```python
from build123d import *

# Parameters (mm, degrees)
SKETCH1_W               = 110
SKETCH1_H               = 70
BOSS_EXTRUDE1_DEPTH     = 5
FILLET2_R               = 5
FILLET3_R               = 5
SKETCH2_W               = 5
SKETCH2_H               = 10
BOSS_EXTRUDE2_DEPTH     = 10
SKETCH3_R               = 1.5
CUT_EXTRUDE1_DEPTH      = 122
SKETCH4_W               = 70
SKETCH4_H               = 10
BOSS_EXTRUDE3_DEPTH     = 10
SKETCH5_R               = 11.5
CUT_EXTRUDE2_DEPTH      = 105
SKETCH6_R               = 1.5
CUT_EXTRUDE3_DEPTH      = 105
CUT_EXTRUDE4_DEPTH      = 55
CUT_EXTRUDE4_DEPTH_BACK = 5
SKETCH9_W               = 90
SKETCH9_H               = 50
CUT_EXTRUDE5_DEPTH      = 55
SKETCH10_R              = 12
CUT_EXTRUDE6_DEPTH      = 109


with BuildPart() as part:
    # Sketch1 → Boss-Extrude1 (new body)
    with BuildSketch(Plane(origin=(0, 0, 0), x_dir=(0, 0, -1), z_dir=(1, 0, 0))):
        with Locations((55, 35)):
            Rectangle(SKETCH1_W, SKETCH1_H)
    extrude(amount=BOSS_EXTRUDE1_DEPTH)

    # Fillet2
    fillet2_edges = [part.edges().sort_by_distance(p)[0] for p in [
        (5, 35, 0),
    ]]
    fillet(fillet2_edges, radius=FILLET2_R - 0.0001)  # a hair under: the kernel refuses the full size

    # Fillet3
    fillet3_edges = [part.edges().sort_by_distance(p)[0] for p in [
        (5, 35, -110),
    ]]
    fillet(fillet3_edges, radius=FILLET3_R - 0.0001)  # a hair under: the kernel refuses the full size

    # Sketch2 → Boss-Extrude2 (add)
    with BuildSketch(Plane.ZY):
        with Locations((-102.5, 65)):
            Rectangle(SKETCH2_W, SKETCH2_H)
        with Locations((-102.5, 5)):
            Rectangle(SKETCH2_W, SKETCH2_H)
        with Locations((-7.5, 5)):
            Rectangle(SKETCH2_W, SKETCH2_H)
        with Locations((-7.5, 65)):
            Rectangle(SKETCH2_W, SKETCH2_H)
    extrude(amount=BOSS_EXTRUDE2_DEPTH)

    # Sketch3 → Cut-Extrude1 (cut)
    with BuildSketch(Plane.XY.offset(-5)):
        with Locations((-5, 65)):
            Circle(SKETCH3_R)
        with Locations((-5, 5)):
            Circle(SKETCH3_R)
    extrude(amount=-CUT_EXTRUDE1_DEPTH, mode=Mode.SUBTRACT)

    # Sketch4 → Boss-Extrude3 (add)
    with BuildSketch(Plane.ZY):
        with Locations((-55, 65)):
            Rectangle(SKETCH4_W, SKETCH4_H)
        with Locations((-55, 5)):
            Rectangle(SKETCH4_W, SKETCH4_H)
    extrude(amount=BOSS_EXTRUDE3_DEPTH)

    # Sketch5 → Cut-Extrude2 (cut)
    with BuildSketch(Plane.XY.offset(-5)):
        with Locations((-17.5, 15)):
            Circle(SKETCH5_R)
    extrude(amount=-CUT_EXTRUDE2_DEPTH, mode=Mode.SUBTRACT)

    # Sketch6 → Cut-Extrude3 (cut)
    with BuildSketch(Plane.XZ):
        with Locations(Location((-3.573842411, -25, 0), (0, 0, 270))):
            Circle(SKETCH6_R)
        with Locations(Location((-3.573842411, -85, 0), (0, 0, 270))):
            Circle(SKETCH6_R)
    extrude(amount=-CUT_EXTRUDE3_DEPTH, mode=Mode.SUBTRACT)

    # Sketch7 → Cut-Extrude4 (cut, two sides: drawn at the far end of the back side and taken through both)
    with BuildSketch(Plane.XZ.offset(-60).offset(-CUT_EXTRUDE4_DEPTH_BACK)):
        Polygon((0.824714328, -27.377540454), (0.68444639, -22.37950835), (-3.71411035, -20.001967897), (-7.972399151, -22.622459546), (-7.832131212, -27.62049165), (-3.433574473, -29.998032103), align=None)
        Polygon((0.654912484, -87.66788906), (0.850994737, -82.671735365), (-3.377760158, -80.003846304), (-7.802597306, -82.33211094), (-7.99867956, -87.328264635), (-3.769924665, -89.996153696), align=None)
    extrude(amount=CUT_EXTRUDE4_DEPTH + CUT_EXTRUDE4_DEPTH_BACK, mode=Mode.SUBTRACT)

    # Sketch9 → Cut-Extrude5 (cut)
    with BuildSketch(Plane.ZY):
        with Locations((-55, 35)):
            Rectangle(SKETCH9_W, SKETCH9_H)
    extrude(amount=-CUT_EXTRUDE5_DEPTH, mode=Mode.SUBTRACT)

    # Sketch10 → Cut-Extrude6 (cut)
    with BuildSketch(Plane.XY.offset(-5)):
        with Locations((-17.5, 15)):
            Circle(SKETCH10_R)
    extrude(amount=-CUT_EXTRUDE6_DEPTH, mode=Mode.SUBTRACT)


solid = part.part
```
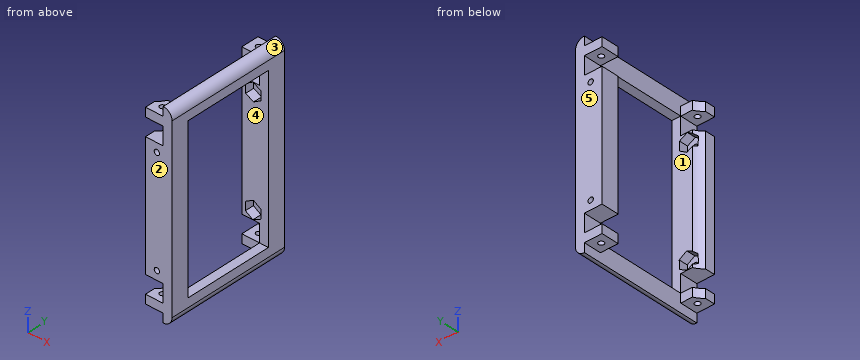
Could you check a few things on this model? Use its own coordinates, in mm. Face numbers are marked on the shaded views. A direction names the side the tool comes from. Round coordinates to 2 decimals unless told otherwise and drop trailing zeros. Write each loop counter-clockwise with the first axis right and the second up, starting at its lowest first coordinate (ties: lowest second). Pieces come first, ordered by that corner, then holes. Notation, with made-up numbers: M 46.5,83.5 L 64.5,83.5 A11 ccw 64.5,93.5 Z; hole C -15.75,28.5 d11. An arc over 180 degrees is marked long. Answer in a Markdown table with one row per item. Add a question column.
Q1. On a 3-axis mill with a long thin cutter (end or side, diameter ignored), from which of +Z, -Z, +X, -X, +Y, -Y can I reach the whole of each face in a straight line? I mean the marked faces 1 and 2. Say none if no direction works.
Q2. If I drill on line 1 (Y direction, x = -5, z = -6); line 2 (Y direction, x = -1.25, z = -32); line 3 (X direction, y = 66, z = -85), over which ranges is the centre line in solid material (lowest first)? Write a range as from..to.
Q3. Will these pins go through, and if not, where does the flat tip stop? pin 1 Ø3 at (x, y) = (-2.5, 4) entering from +Z; pin 2 Ø4 at (x, y) = (-5, 65) entering from -Z.
Q4. Imagine slicing it at D-D (z = -103). Please give me the cut outline in (x, y).
Q5. If we mould it in two halves opening along Z, with no side actions, what happens to the marked faces 3, 4 and 5? For each: +Z half, -Z half, draft (parallel to the pull), parting line (faces both ways), or undercut.
Q6. Imagine slicing it at A-A (z = -12). Please give me the cut outline in (x, y).
Q7. Imagine slicing it at C-C (z = -85). Please give me the cut outline in (x, y), then the cut area to 3 significant figures.
Values:
| question | item | result |
|---|---|---|
| 1 | face 1 | +X, -X |
| 1 | face 2 | +Z, -Z, +X, -X, -Y |
| 2 | line 1 | 0..3.5, 6.5..10, 60..63.5, 66.5..70 |
| 2 | line 2 | 0..10, 60..70 |
| 2 | line 3 | -10..-5.07, -2.07..5 |
| 3 | pin 1 | z = -5 |
| 3 | pin 2 | z = -105 |
| 4 | outline | M -10,0 L 5,0 L 5,70 L -10,70 L -10,60 L 0,60 L 0,10 L -6.59,10 A12 cw -10,5.63 Z; hole C -5,5 d3; hole C -5,65 d3 |
| 5 | face 3 | +Z half |
| 5 | face 4 | undercut |
| 5 | face 5 | draft |
| 6 | outline | M 0,0 L 5,0 L 5,10 L 0,10 Z; M 0,60 L 5,60 L 5,70 L 0,70 Z |
| 7 | outline | M -10,0 L -5.07,0 L -5.07,5 L -7.91,5 L -7.91,7.79 A12 cw -10,5.63 Z; M -10,60 L -7.91,60 L -7.91,65 L -5.07,65 L -5.07,70 L -10,70 Z; M -2.07,0 L 5,0 L 5,10 L 0.76,10 L 0.76,5 L -2.07,5 Z; M -2.07,65 L 0.76,65 L 0.76,60 L 5,60 L 5,70 L -2.07,70 Z |
| 7 | area | 176 mm^2 |
